Could you check a few things on this model? Use its own coordinates, in mm. Coordinates: 2 decimals unless noted, no trailing zeros. Loops run counter-clockwise (first coordinate to the right, second up) from the corner with the lowest first, then second, coordinate; pieces in that order, holes last. Notation, with made-up numbers: (-10.75, -27.75) - (21.25, -27.75) arc R14 ccw to (21.25, -23.75) - close; hole circle Ø10 at (-32.5, -16). An arc over 180 degrees is marked (long way). Use CSV: the item, a comma, the result in double quotes.
from build123d import *

# Parameters (mm, degrees)
BOX433_W                     = 6
BOX433_H                     = 8
BOX433_DEPTH                 = 2
BOX433_PLACEMENT_ANGLE       = 45
BOX435_W                     = 6
BOX435_H                     = 8
BOX435_DEPTH                 = 2
BOX426_W                     = 6
BOX426_H                     = 8
BOX426_DEPTH                 = 2
BOX438_W                     = 6
BOX438_H                     = 8
BOX438_DEPTH                 = 2
BOX438_PLACEMENT_ANGLE       = 135
BOX436_W                     = 6
BOX436_H                     = 8
BOX436_DEPTH                 = 2
BOX440_W                     = 6
BOX440_H                     = 8
BOX440_DEPTH                 = 2
BOX440_PLACEMENT_ANGLE       = 225
BOX429_W                     = 6
BOX429_H                     = 8
BOX429_DEPTH                 = 2
BOX439_W                     = 6
BOX439_H                     = 8
BOX439_DEPTH                 = 2
BOX439_PLACEMENT_ANGLE       = 45
COMPOUND873_PLACEMENT_ANGLE  = 22.5
CYLINDER1120_R               = 1.5
CYLINDER1120_DEPTH           = 12
CYLINDER1120_PLACEMENT_ANGLE = 45
CYLINDER1128_R               = 1.5
CYLINDER1128_DEPTH           = 12
CYLINDER1126_R               = 1.5
CYLINDER1126_DEPTH           = 12
CYLINDER1126_PLACEMENT_ANGLE = 135
CYLINDER1125_R               = 1.5
CYLINDER1125_DEPTH           = 12
CYLINDER1127_R               = 1.5
CYLINDER1127_DEPTH           = 12
CYLINDER1127_PLACEMENT_ANGLE = 225
CYLINDER1124_R               = 1.5
CYLINDER1124_DEPTH           = 12
CYLINDER1119_R               = 1.5
CYLINDER1119_DEPTH           = 12
CYLINDER1119_PLACEMENT_ANGLE = 45
CYLINDER1122_R               = 1.5
CYLINDER1122_DEPTH           = 12
COMPOUND874_PLACEMENT_ANGLE  = 22.5
CYLINDER1117_R               = 3.5
CYLINDER1117_DEPTH           = 20
TUBE101_R                    = 46
TUBE101_R_2                  = 36
TUBE101_DEPTH                = 1


with BuildPart() as krychle433:
    # Box433 → Box433 (new body)
    with BuildSketch(Plane.XY):
        with Locations((3, 4)):
            Rectangle(BOX433_W, BOX433_H)
    extrude(amount=BOX433_DEPTH)


with BuildPart() as krychle433_1:
    # Box433 placement: moved
    add(krychle433.part.moved(Location((30.405592, -34.648232, 33))).rotate(Axis((30.405592, -34.648232, 33), (0, 0, 1)), BOX433_PLACEMENT_ANGLE))


with BuildPart() as krychle435:
    # Box435 → Box435 (new body)
    with BuildSketch(Plane(origin=(46, -3, 33), x_dir=(0, 1, 0), z_dir=(0, 0, 1))):
        with Locations((3, 4)):
            Rectangle(BOX435_W, BOX435_H)
    extrude(amount=BOX435_DEPTH)


with BuildPart() as krychle426:
    # Box426 → Box426 (new body)
    with BuildSketch(Plane(origin=(-3, -46, 33), x_dir=(1, 0, 0), z_dir=(0, 0, 1))):
        with Locations((3, 4)):
            Rectangle(BOX426_W, BOX426_H)
    extrude(amount=BOX426_DEPTH)


with BuildPart() as krychle438:
    # Box438 → Box438 (new body)
    with BuildSketch(Plane.XY):
        with Locations((3, 4)):
            Rectangle(BOX438_W, BOX438_H)
    extrude(amount=BOX438_DEPTH)


with BuildPart() as krychle438_1:
    # Box438 placement: moved
    add(krychle438.part.moved(Location((34.648232, 30.405592, 33))).rotate(Axis((34.648232, 30.405592, 33), (0, 0, 1)), BOX438_PLACEMENT_ANGLE))


with BuildPart() as krychle436:
    # Box436 → Box436 (new body)
    with BuildSketch(Plane(origin=(3, 46, 33), x_dir=(-1, 0, 0), z_dir=(0, 0, 1))):
        with Locations((3, 4)):
            Rectangle(BOX436_W, BOX436_H)
    extrude(amount=BOX436_DEPTH)


with BuildPart() as krychle440:
    # Box440 → Box440 (new body)
    with BuildSketch(Plane.XY):
        with Locations((3, 4)):
            Rectangle(BOX440_W, BOX440_H)
    extrude(amount=BOX440_DEPTH)


with BuildPart() as krychle440_1:
    # Box440 placement: moved
    add(krychle440.part.moved(Location((-30.405592, 34.648232, 33))).rotate(Axis((-30.405592, 34.648232, 33), (0, 0, 1)), BOX440_PLACEMENT_ANGLE))


with BuildPart() as krychle429:
    # Box429 → Box429 (new body)
    with BuildSketch(Plane(origin=(-46, 3, 33), x_dir=(0, -1, 0), z_dir=(0, 0, 1))):
        with Locations((3, 4)):
            Rectangle(BOX429_W, BOX429_H)
    extrude(amount=BOX429_DEPTH)


with BuildPart() as compound873:
    # Box439 → Box439 (new body)
    with BuildSketch(Plane.XY):
        with Locations((3, 4)):
            Rectangle(BOX439_W, BOX439_H)
    extrude(amount=BOX439_DEPTH)


with BuildPart() as compound873_1:
    # Box439 placement: moved
    add(compound873.part.moved(Location((-34.648232, -30.405592, 33))).rotate(Axis((-34.648232, -30.405592, 33), (0, 0, -1)), BOX439_PLACEMENT_ANGLE))

    # Compound873: union Krychle433, Krychle435, Krychle426, Krychle438, Krychle436, Krychle440, Krychle429
    add(krychle433_1.part)
    add(krychle435.part)
    add(krychle426.part)
    add(krychle438_1.part)
    add(krychle436.part)
    add(krychle440_1.part)
    add(krychle429.part)


with BuildPart() as compound873_2:
    # Compound873 placement: moved
    add(compound873_1.part.moved(Location((0, 0, 7))).rotate(Axis((0, 0, 7), (0, 0, 1)), COMPOUND873_PLACEMENT_ANGLE))


with BuildPart() as obj1:
    # Cylinder1120 → Cylinder1120 (new body)
    with BuildSketch(Plane.XY):
        Circle(CYLINDER1120_R)
    extrude(amount=CYLINDER1120_DEPTH)


with BuildPart() as obj1_1:
    # Cylinder1120 placement: moved
    add(obj1.part.moved(Location((29.698485, -29.698485, 33.5))).rotate(Axis((29.698485, -29.698485, 33.5), (0, 0, 1)), CYLINDER1120_PLACEMENT_ANGLE))


with BuildPart() as obj2:
    # Cylinder1128 → Cylinder1128 (new body)
    with BuildSketch(Plane(origin=(42, 0, 33.5), x_dir=(0, 1, 0), z_dir=(0, 0, 1))):
        Circle(CYLINDER1128_R)
    extrude(amount=CYLINDER1128_DEPTH)


with BuildPart() as obj3:
    # Cylinder1126 → Cylinder1126 (new body)
    with BuildSketch(Plane.XY):
        Circle(CYLINDER1126_R)
    extrude(amount=CYLINDER1126_DEPTH)


with BuildPart() as obj3_1:
    # Cylinder1126 placement: moved
    add(obj3.part.moved(Location((29.698485, 29.698485, 33.5))).rotate(Axis((29.698485, 29.698485, 33.5), (0, 0, 1)), CYLINDER1126_PLACEMENT_ANGLE))


with BuildPart() as obj4:
    # Cylinder1125 → Cylinder1125 (new body)
    with BuildSketch(Plane(origin=(0, 42, 33.5), x_dir=(-1, 0, 0), z_dir=(0, 0, 1))):
        Circle(CYLINDER1125_R)
    extrude(amount=CYLINDER1125_DEPTH)


with BuildPart() as obj5:
    # Cylinder1127 → Cylinder1127 (new body)
    with BuildSketch(Plane.XY):
        Circle(CYLINDER1127_R)
    extrude(amount=CYLINDER1127_DEPTH)


with BuildPart() as obj5_1:
    # Cylinder1127 placement: moved
    add(obj5.part.moved(Location((-29.698485, 29.698485, 33.5))).rotate(Axis((-29.698485, 29.698485, 33.5), (0, 0, 1)), CYLINDER1127_PLACEMENT_ANGLE))


with BuildPart() as obj6:
    # Cylinder1124 → Cylinder1124 (new body)
    with BuildSketch(Plane(origin=(-42, 0, 33.5), x_dir=(0, -1, 0), z_dir=(0, 0, 1))):
        Circle(CYLINDER1124_R)
    extrude(amount=CYLINDER1124_DEPTH)


with BuildPart() as obj7:
    # Cylinder1119 → Cylinder1119 (new body)
    with BuildSketch(Plane.XY):
        Circle(CYLINDER1119_R)
    extrude(amount=CYLINDER1119_DEPTH)


with BuildPart() as obj7_1:
    # Cylinder1119 placement: moved
    add(obj7.part.moved(Location((-29.698485, -29.698485, 33.5))).rotate(Axis((-29.698485, -29.698485, 33.5), (0, 0, -1)), CYLINDER1119_PLACEMENT_ANGLE))


with BuildPart() as compound874:
    # Cylinder1122 → Cylinder1122 (new body)
    with BuildSketch(Plane(origin=(0, -42, 33.5), x_dir=(1, 0, 0), z_dir=(0, 0, 1))):
        Circle(CYLINDER1122_R)
    extrude(amount=CYLINDER1122_DEPTH)

    # Compound874: union obj1, obj2, obj3, obj4, obj5, obj6, obj7
    add(obj1_1.part)
    add(obj2.part)
    add(obj3_1.part)
    add(obj4.part)
    add(obj5_1.part)
    add(obj6.part)
    add(obj7_1.part)


with BuildPart() as compound874_1:
    # Compound874 placement: moved
    add(compound874.part.moved(Location((0, 0, 4))).rotate(Axis((0, 0, 4), (0, 0, 1)), COMPOUND874_PLACEMENT_ANGLE))


with BuildPart() as obj8:
    # Cylinder1117 → Cylinder1117 (new body)
    with BuildSketch(Plane(origin=(-46.4, 0, 34), x_dir=(1, 0, 0), z_dir=(0, 0, 1))):
        Circle(CYLINDER1117_R)
    extrude(amount=CYLINDER1117_DEPTH)


with BuildPart() as cut422:
    # Tube101 → Tube101 (new body)
    with BuildSketch(Plane.XY.offset(45)):
        Circle(TUBE101_R)
        Circle(TUBE101_R_2, mode=Mode.SUBTRACT)
    extrude(amount=TUBE101_DEPTH)

    # Cut424: cut obj8
    add(obj8.part, mode=Mode.SUBTRACT)

    # Cut425: cut Compound874
    add(compound874_1.part, mode=Mode.SUBTRACT)

    # Cut422: cut Compound873
    add(compound873_2.part, mode=Mode.SUBTRACT)


solid = cut422.part
(1) Will this pin go through, and if not, where does the flat tip stop? pin 1 (1.8 mm diameter, centred on x = -16.07, y = 38.8, fed in from +Z).
Computed:
pin 1,"passes through"
(2) Suppose I cut it at C-C (z = 45.45). State how many separate pieces and enclosed holes the cut face has, plus the area to 3 significant figures.
Computed:
separate pieces,"1"
enclosed holes,"9"
area,"2,500 mm²"
(3) Suppose I cut it at A-A (x = 0). Write out the boundary of the cut face in (y, z).
Computed:
outline,"(-46, 45) - (-36, 45) - (-36, 46) - (-46, 46) - close; (36, 45) - (46, 45) - (46, 46) - (36, 46) - close"
(4) Please list where these lines run through material, in increasing order: line 1 (Y direction, x = 15, z = 45.85); line 2 (X direction, y = 8.5, z = 45.6); line 3 (X direction, y = -11.5, z = 45.9).
Computed:
line 1,"y = -43.49 to -39.85, -37.75 to -32.73, 32.73 to 37.75, 39.85 to 43.49"
line 2,"x = -45.21 to -34.98, 34.98 to 45.21"
line 3,"x = -44.54 to -34.11, 34.11 to 44.54"
(5) Suppose I cut it at B-B (y = 0). Write out the boundary of the cut face in (x, z), plus the area to 3 significant figures.
Computed:
outline,"(-42.9, 45) - (-36, 45) - (-36, 46) - (-42.9, 46) - close; (36, 45) - (46, 45) - (46, 46) - (36, 46) - close"
area,"16.9 mm²"
(6) Thinking about a two-plate mould opening in Y: for faces 1 (the face through (45.958, -1.974, 45.493)), 2 (the face through (37.943, -14.844, 45.493)), 3 (the face through (14.844, 37.943, 45.493)), 4 (the face through (-27.4, -23.6, 45)), which applies, +Y half, -Y half, draft (parallel to the pull), parting line (faces both ways), or undercut?
Computed:
face 1,"parting line"
face 2,"undercut"
face 3,"undercut"
face 4,"draft"
